Here's the drawing with two shaded views (mm, measured from the low corner). I have some questions. Give positions to 0.01 mm unless a question says otherwise; leave off trailing zeros. Write each loop counter-clockwise with the first axis right and the second up, starting at its lowest first coordinate (ties: lowest second). Pieces come first, ordered by that corner, then holes. Notation, with made-up numbers: (35, 50.25) - (46, 50.25) arc R27 cw to (46, 89.25) - close; hole circle Ø2 at (-8, 71.5). An arc over 180 degrees is marked (long way). Write item = value, one per line.
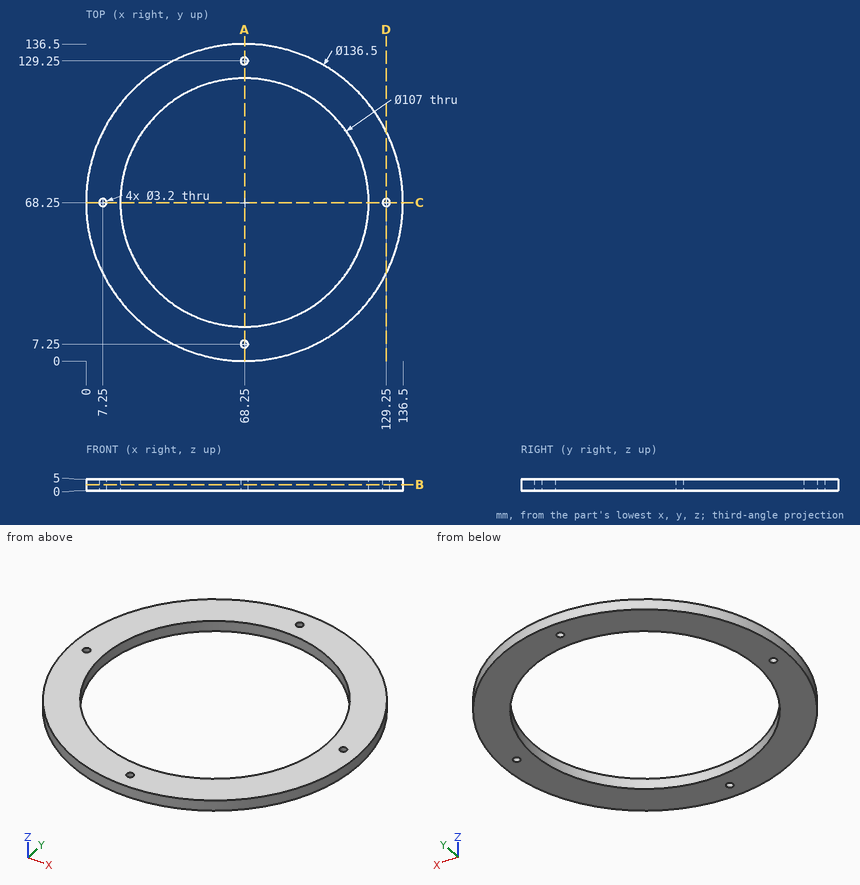
1. If we section it at D-D, the plane x = 129.25: Please give me the cut outline in (y, z).
Filled sheet:
outline = (37.64, 0) - (66.65, 0) - (66.65, 5) - (37.64, 5) - close; (69.85, 0) - (98.86, 0) - (98.86, 5) - (69.85, 5) - close
2. I need wall thicknesses on line 1 (Y direction, x = 68.25, z = 3.7); line 2 (Y direction, x = 7.25, z = 3.55); line 3 (Y direction, x = 22, z = 2.85). Which ranges of each line are inside material? Lowest first, please.
Filled sheet:
line_1 = 0 to 5.65, 8.85 to 14.75, 121.75 to 127.65, 130.85 to 136.5
line_2 = 37.64 to 66.65, 69.85 to 98.86
line_3 = 18.06 to 41.36, 95.14 to 118.44
3. For pin 1 (6 mm diameter, centred on x = 68.5, y = 16.5, fed in from +Z); pin 2 (2.5 mm diameter, centred on x = 7.25, y = 68.25, fed in from +Z); pin 3 (1 mm diameter, centred on y = 49, z = 2.5, fed in from +X); pin 4 (1.5 mm diameter, centred on y = 48.5, z = 0.5, fed in from +X), each with a flat end and sliding along its axis, tell me the tip position at first contact or that it passes through.
Filled sheet:
pin_1 = 5
pin_2 = through
pin_3 = 133.87
pin_4 = 133.8
4. If we section it at A-A, the plane x = 68.25: Please give me the cut outline in (y, z).
Filled sheet:
outline = (0, 0) - (5.65, 0) - (5.65, 5) - (0, 5) - close; (8.85, 0) - (14.75, 0) - (14.75, 5) - (8.85, 5) - close; (121.75, 0) - (127.65, 0) - (127.65, 5) - (121.75, 5) - close; (130.85, 0) - (136.5, 0) - (136.5, 5) - (130.85, 5) - close
5. If we section it at B-B, the plane z = 2.55: Please give me the cut outline in (x, y), and give its area (3 significant figures).
Filled sheet:
outline = circle Ø136.5 at (68.25, 68.25); hole circle Ø3.2 at (7.25, 68.25); hole circle Ø107 at (68.25, 68.25); hole circle Ø3.2 at (68.25, 7.25); hole circle Ø3.2 at (68.25, 129.25); hole circle Ø3.2 at (129.25, 68.25)
area = 5,610 mm2
